Answer from the drawing. Dimensions are ordinates in mm from the lowest x, y and z of the part. A direction names the side the tool comes from. Give positions to 0.01 mm unless a question says otherwise; leave off trailing zeros. Write each loop counter-clockwise with the first axis right and the second up, starting at its lowest first coordinate (ties: lowest second). Pieces come first, ordered by that corner, then holes.
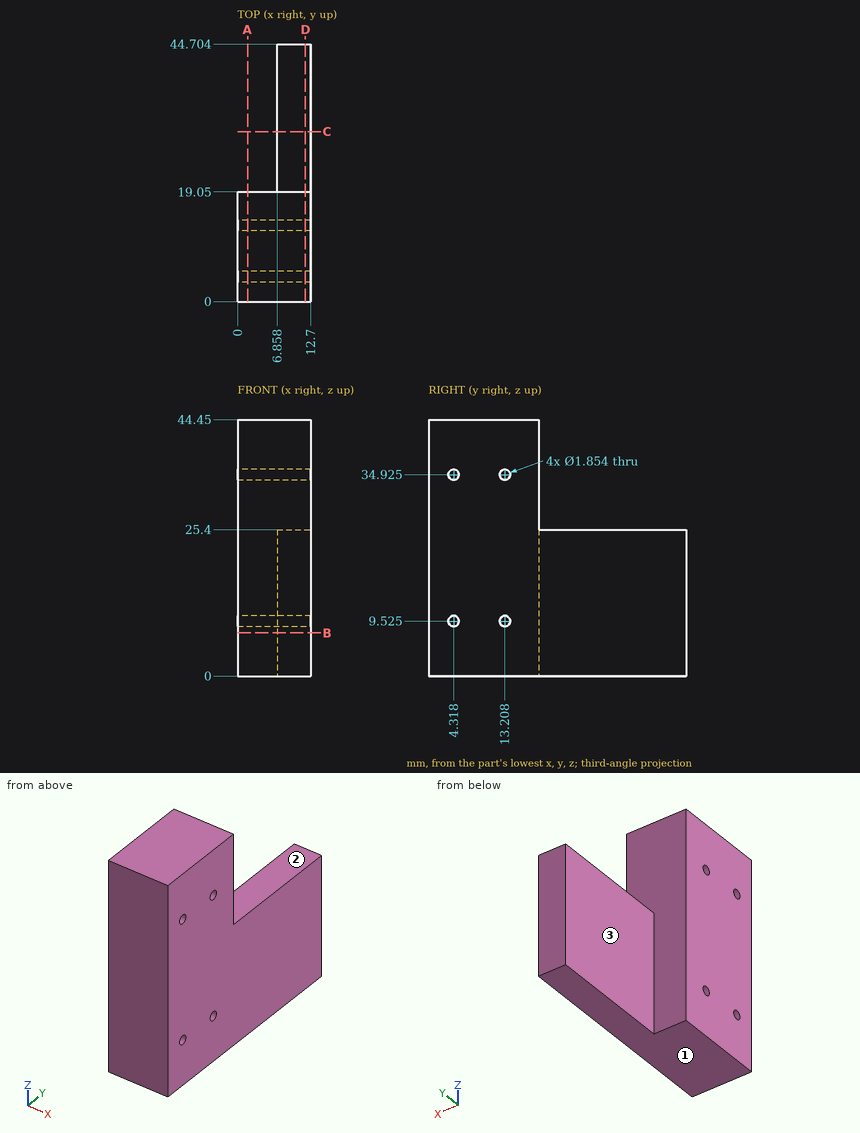
Item 1: A cutting plane is placed at D-D, the plane x = 11.75. Give the vertices of the cut face in (y, z) (3 decimals).
Conclusion:
outline: (0, 0) - (44.704, 0) - (44.704, 25.4) - (19.05, 25.4) - (19.05, 44.45) - (0, 44.45) - close; hole circle Ø1.854 at (4.318, 9.525); hole circle Ø1.854 at (4.318, 34.925); hole circle Ø1.854 at (13.208, 9.525); hole circle Ø1.854 at (13.208, 34.925)
Item 2: Which of the six approach directions +Z, -Z, +X, -X, +Y, -Y give full straight-line access (tool end or side, diameter ignored) to the marked faces 1, 2 and 3?
Conclusion:
face 1: -Z, +X, -X, +Y, -Y
face 2: +Z, +X, -X, +Y
face 3: +Z, -Z, -X, +Y
Item 3: Consider probe 1 along X at (y, z) = (32, 6); probe 2 along Y at (x, z) = (6, 25); probe 3 along Z at (x, y) = (9.75, 27). Determine where each line is inside the solid, lowest interval first.
Conclusion:
probe 1: x = 6.86 to 12.7
probe 2: y = 0 to 19.05
probe 3: z = 0 to 25.4
Item 4: Each of these flat-tipped pins is pushed along its axis until it touches: P1, Ø2, axis at y = 13.208, z = 9.525, coming from the +X side; P2, Ø6.5, axis at x = 8.5, y = 25.5, coming from the +Z side; P3, Ø5, axis at x = 1.5, z = 10, coming from the +Y side; P4, Ø1.7, axis at y = 4.318, z = 34.925, coming from the +X side. Where does it stop, or does it pass through?
Conclusion:
P1: stops at x = 12.7
P2: stops at z = 25.4
P3: stops at y = 19.05
P4: passes through
Item 5: A cutting plane is placed at A-A, the plane x = 1.75. Give the vertices of the cut face in (y, z) (3 decimals), plus the area to 3 significant figures.
Conclusion:
outline: (0, 0) - (19.05, 0) - (19.05, 44.45) - (0, 44.45) - close; hole circle Ø1.854 at (4.318, 9.525); hole circle Ø1.854 at (4.318, 34.925); hole circle Ø1.854 at (13.208, 9.525); hole circle Ø1.854 at (13.208, 34.925)
area: 836 mm2
Item 6: A cutting plane is placed at B-B, the plane z = 7.5. Give the vertices of the cut face in (x, y).
Conclusion:
outline: (0, 0) - (12.7, 0) - (12.7, 44.7) - (6.86, 44.7) - (6.86, 19.05) - (0, 19.05) - close
Item 7: A cutting plane is placed at C-C, the plane y = 29.5. Give the vertices of the cut face in (x, z).
Conclusion:
outline: (6.86, 0) - (12.7, 0) - (12.7, 25.4) - (6.86, 25.4) - close
